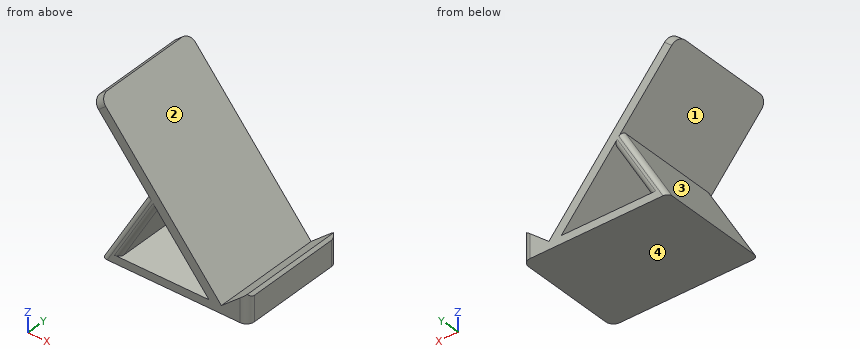
```python
from build123d import *

# Parameters (mm, degrees)
PAD_DEPTH   = 70
FILLET_R    = 6
FILLET001_R = 5
FILLET002_R = 3


with BuildPart() as part:
    # Sketch → Pad (new body)
    with BuildSketch(Plane.XZ):
        Polygon((0, 0), (0, 16), (-1.557161, 17.855752), (-16.87805, 5), (-94.012563, 96.925333), (-98.60883, 93.068608), (-63.255511, 50.936163), (-92.663519, 0), align=None)
        Polygon((-58.11321, 44.807808), (-24.688255, 4.973497), (-81.11156, 4.973497), align=None, mode=Mode.SUBTRACT)
    extrude(amount=PAD_DEPTH)

    # Fillet
    fillet_edges = [part.edges().sort_by_distance(p)[0] for p in [
        (-96.310696, -70, 94.99697),
        (-96.310696, 0, 94.99697),
    ]]
    fillet(fillet_edges, radius=FILLET_R)

    # Fillet001
    fillet001_edges = [part.edges().sort_by_distance(p)[0] for p in [
        (0, -70, 8),
        (0, 0, 8),
    ]]
    fillet(fillet001_edges, radius=FILLET001_R)

    # Fillet002
    fillet002_edges = [part.edges().sort_by_distance(p)[0] for p in [
        (-69.612385, -70, 24.890652),
        (-77.959515, -70, 25.468082),
        (-77.959515, 0, 25.468082),
        (-69.612385, 0, 24.890652),
    ]]
    fillet(fillet002_edges, radius=FILLET002_R)


solid = part.part
```
Can you work these out from the model? Positions are in its coordinate system, mm. Face numbers are marked on the shaded views. Round coordinates to 2 decimals unless told otherwise and drop trailing zeros. Order: outer loops, then holes, each group sorted by start corner. A loop starts at its lowest first (then second) coordinate and runs counter-clockwise, first axis right, second up.
(1) If we section it at B-B (x = -55): Please give me the cut outline in (y, z).
Results are:
outline: (-70, 0) - (0, 0) - (0, 4.97) - (-70, 4.97) - close; (-70, 41.1) - (0, 41.1) - (0, 50.43) - (-70, 50.43) - close
(2) If we section it at C-C (x = -71): Count the separate pieces of the cut face and the enclosed holes in it, plus the area to 3 significant figures.
Results are:
separate pieces: 3
enclosed holes: 0
area: 2,040 mm2
(3) If we section it at A-A (y = -58.5): Please give me the cut outline in (x, z).
Results are:
outline: (-98.61, 93.07) - (-63.26, 50.94) - (-92.66, 0) - (0, 0) - (0, 16) - (-1.56, 17.86) - (-16.88, 5) - (-94.01, 96.93) - close; hole (-81.11, 4.97) - (-24.69, 4.97) - (-58.11, 44.81) - close
(4) If I drill on L1, parallel to X at y = -13, z = 26; L2, parallel to X at y = -30.5, z = 38; L3, parallel to Z at x = -47.5, y = -44.5, over which ranges is the centre line in solid material (lowest first)?
Results are:
L1: x = -77.65 to -68.97, -42.33 to -34.5
L2: x = -70.72 to -62.04, -52.4 to -44.57
L3: z = 0 to 4.97, 32.16 to 41.49
(5) If we section it at D-D (z = 83.5): Please give me the cut outline in (x, y), plus the area to 3 significant figures.
Results are:
outline: (-90.58, -70) - (-82.75, -70) - (-82.75, 0) - (-90.58, 0) - close
area: 548 mm2
(6) We'd pull the mould along Z, two halves only. Please class the marked faces 1, 2, 3 and 4: +Z half, -Z half, draft (parallel to the pull), parting line (faces both ways), or undercut.
Results are:
face 1: undercut
face 2: +Z half
face 3: undercut
face 4: -Z half
(7) I'm going to push flat-ended pins straight in: pin 1 (12 mm diameter, centred on x = -20, z = 23.5, fed in from -Y); pin 2 (4 mm diameter, centred on y = -48.5, z = 83, fed in from +X); pin 3 (18 mm diameter, centred on x = -50, y = -35.5, fed in from +Z); pin 4 (10 mm diameter, centred on x = -56, y = -31, fed in from -Z). Where does each tip first touch, or does it pass through?
Results are:
pin 1: passes through
pin 2: stops at x = -80.65
pin 3: stops at z = 55.2
pin 4: stops at z = 0
